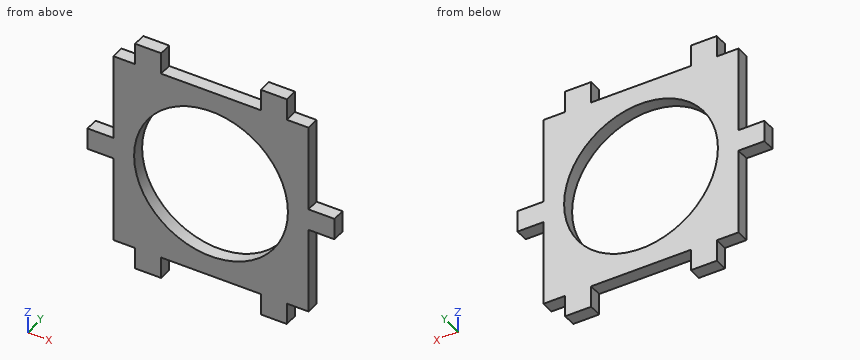
```python
from build123d import *

# Parameters (mm, degrees)
CROQUIS1_W              = 45
CROQUIS1_H              = 45
CROQUIS1_R              = 17.75
CROQUIS1_W_2            = 6
CROQUIS1_H_2            = 5
SALIENTE_EXTRUIR1_DEPTH = 3
CROQUIS1_3_W            = 6
CROQUIS1_3_H            = 5
SALIENTE_EXTRUIR2_DEPTH = 3


with BuildPart() as part:
    # Croquis1 → Saliente-Extruir1 (new body)
    with BuildSketch(Plane(origin=(0, 0, 0), x_dir=(1, 0, 0), z_dir=(0, 1, 0))):
        Rectangle(CROQUIS1_W, CROQUIS1_H)
        Circle(CROQUIS1_R, mode=Mode.SUBTRACT)
        with Locations((-14.5, 25)):
            Rectangle(CROQUIS1_W_2, CROQUIS1_H_2)
        with Locations((14.5, 25)):
            Rectangle(CROQUIS1_W_2, CROQUIS1_H_2)
        with Locations((-14.5, -25)):
            Rectangle(CROQUIS1_W_2, CROQUIS1_H_2)
        with Locations((14.5, -25)):
            Rectangle(CROQUIS1_W_2, CROQUIS1_H_2)
    extrude(amount=SALIENTE_EXTRUIR1_DEPTH)

    # Croquis1_3 → Saliente-Extruir2 (add)
    with BuildSketch(Plane(origin=(0, 0, 0), x_dir=(1, 0, 0), z_dir=(0, 1, 0))):
        with Locations((-25.5, 0)):
            Rectangle(CROQUIS1_3_W, CROQUIS1_3_H)
        with Locations((25.5, 0)):
            Rectangle(CROQUIS1_3_W, CROQUIS1_3_H)
    extrude(amount=SALIENTE_EXTRUIR2_DEPTH)


solid = part.part
```
CAD build for the part. Positions are in the model's coordinates, mm. Round coordinates to 2 decimals unless told otherwise and drop trailing zeros. Order: outer loops, then holes, each group sorted by start corner. A loop starts at its lowest first (then second) coordinate and runs counter-clockwise, first axis right, second up.
Q1. Slice it at D-D (x = 20.5). Write the cut outline in (y, z).
Q2. Slice it at C-C (z = 0). Write the cut outline in (x, y).
Q3. Drop flat-ended pins along their axis: pin 1 (0.9 mm diameter, centred on x = -19.5, y = 1, fed in from -Z); pin 2 (1 mm diameter, centred on y = 1.5, z = -12, fed in from -X); pin 3 (0.9 mm diameter, centred on y = 1, z = 10, fed in from +X); pin 4 (8 mm diameter, centred on x = -11, z = 14, fed in from -Y). Give the stop position or say it passes through.
Q4. Wall check: L1, parallel to X at y = 0.8, z = 0; L2, parallel to Z at x = 0, y = 1.4; L3, parallel to X at y = 2.6, z = 23.5. Give the ranges that are in metal, low to high.
Q5. Slice it at B-B (x = 0). Write the cut outline in (y, z), and give its area (3 significant figures).
Results below:
1. outline: (0, -22.5) - (3, -22.5) - (3, 22.5) - (0, 22.5) - close
2. outline: (-28.5, 0) - (-17.75, 0) - (-17.75, 3) - (-28.5, 3) - close; (17.75, 0) - (28.5, 0) - (28.5, 3) - (17.75, 3) - close
3. pin 1: stops at z = -22.5
3. pin 2: stops at x = -22.5
3. pin 3: stops at x = 22.5
3. pin 4: stops at y = 0
4. L1: x = -28.5 to -17.75, 17.75 to 28.5
4. L2: z = -22.5 to -17.75, 17.75 to 22.5
4. L3: x = -17.5 to -11.5, 11.5 to 17.5
5. outline: (0, -22.5) - (3, -22.5) - (3, -17.75) - (0, -17.75) - close; (0, 17.75) - (3, 17.75) - (3, 22.5) - (0, 22.5) - close
5. area: 28.5 mm2
